Verification items for the finished model (mm, model axes). Face numbers are marked on the shaded views. Round coordinates to 2 decimals unless told otherwise and drop trailing zeros. Loops run counter-clockwise (first coordinate to the right, second up) from the corner with the lowest first, then second, coordinate; pieces in that order, holes last. Notation, with made-up numbers: (47.5, -24.5) - (98.5, -24.5) arc R31 ccw to (98.5, 4.5) - close; hole circle Ø7 at (-21.75, 87). An arc over 180 degrees is marked (long way). Use a Markdown table: item, result. Add a question column.
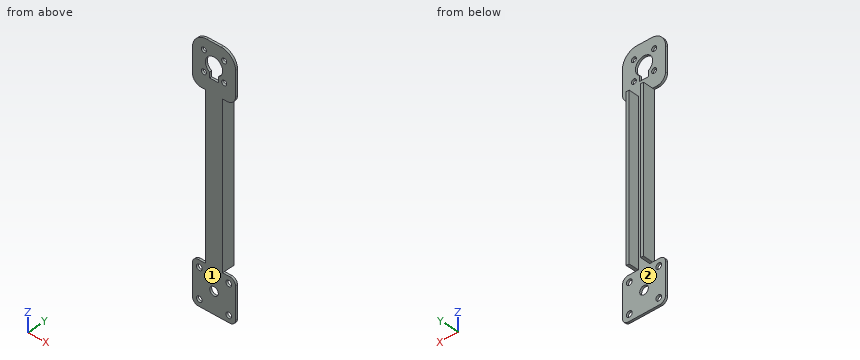
```python
from build123d import *

# Parameters (mm, degrees)
SKETCH_2_W           = 30
SKETCH_2_H           = 31
SKETCH_2_R           = 3
EXTRUDE_1_DEPTH      = 1.5
SKETCH_4_W           = 30
SKETCH_4_H           = 137
SKETCH_4_R           = 1.75
SKETCH_4_R_2         = 6
EXTRUDE_2_DEPTH      = 1.5
SKETCH_5_W           = 6
SKETCH_5_H           = 6
CUT_EXTRUDE_1_DEPTH  = 161.708587201
FILLET_7_R           = 10
CUT_EXTRUDE_2_DEPTH  = 161.708587201
FILLET_10_R          = 6
EXTRUDE_START        = -1.5
SKETCH_7_W           = 30
SKETCH_7_H           = 30
SKETCH_7_R           = 3
SKETCH_7_R_2         = 2
EXTRUDE_3_DEPTH      = 1.5
FILLET_12_R          = 4
EXTRUDE_4_DEPTH      = 7
EXTRUDE_4_DEPTH_BACK = 1.5
SKETCH_8_W           = 2
SKETCH_8_H           = 112


with BuildPart() as part:
    # 草图2 → 凸台-拉伸1 (new body)
    with BuildSketch(Plane(origin=(0, 0, 0), x_dir=(1, 0, 0), z_dir=(0, 1, 0))):
        with Locations((0, -7.5)):
            Rectangle(SKETCH_2_W, SKETCH_2_H)
        with Locations(Location((0, 0, 0), (0, 0, 270))):
            Circle(SKETCH_2_R, mode=Mode.SUBTRACT)
    extrude(amount=EXTRUDE_1_DEPTH)

    # 草图4 → 凸台-拉伸2 (add)
    with BuildSketch(Plane(origin=(0, 1.5, 0), x_dir=(1, 0, 0), z_dir=(0, 1, 0))):
        with Locations((0, -91.5)):
            Rectangle(SKETCH_4_W, SKETCH_4_H)
        with Locations(Location((7.071067812, -137.928932188, 0), (0, 0, 270))):
            Circle(SKETCH_4_R, mode=Mode.SUBTRACT)
        with Locations(Location((-7.071067812, -152.071067812, 0), (0, 0, 270))):
            Circle(SKETCH_4_R, mode=Mode.SUBTRACT)
        with Locations(Location((-7.071067812, -137.928932188, 0), (0, 0, 270))):
            Circle(SKETCH_4_R, mode=Mode.SUBTRACT)
        with Locations(Location((7.071067812, -152.071067812, 0), (0, 0, 270))):
            Circle(SKETCH_4_R, mode=Mode.SUBTRACT)
        with Locations(Location((0, -145, 0), (0, 0, 270))):
            Circle(SKETCH_4_R_2, mode=Mode.SUBTRACT)
    extrude(amount=-EXTRUDE_2_DEPTH)

    # 草图5 → 切除-拉伸1 (cut, through all)
    with BuildSketch(Plane(origin=(0, 1.5, 0), x_dir=(1, 0, 0), z_dir=(0, 1, 0))):
        with Locations((0, -139)):
            Rectangle(SKETCH_5_W, SKETCH_5_H)
    extrude(amount=-CUT_EXTRUDE_1_DEPTH, mode=Mode.SUBTRACT)

    # 圆角7
    fillet_7_edges = [part.edges().sort_by_distance(p)[0] for p in [
        (-15, 0.75, 160),
        (15, 0.75, 160),
    ]]
    fillet(fillet_7_edges, radius=FILLET_7_R)

    # 草图6 → 切除-拉伸2 (cut, through all)
    with BuildSketch(Plane(origin=(0, 1.5, 0), x_dir=(1, 0, 0), z_dir=(0, 1, 0))):
        Polygon((-8, 8), (-8, -8), (-4, -8), (-4, -127), (-8, -127), (-15, -127), (-15, 8), align=None)
        Polygon((15, 8), (8, 8), (8, -8), (4, -8), (4, -127), (8, -127), (15, -127), align=None)
    extrude(amount=-CUT_EXTRUDE_2_DEPTH, mode=Mode.SUBTRACT)

    # 圆角10
    fillet_10_edges = [part.edges().sort_by_distance(p)[0] for p in [
        (-15, 0.75, 127),
        (15, 0.75, 127),
    ]]
    fillet(fillet_10_edges, radius=FILLET_10_R)

    # 草图7 → 凸台-拉伸3 (add)
    with BuildSketch(Plane(origin=(0, 1.5, 0), x_dir=(1, 0, 0), z_dir=(0, 1, 0)).offset(EXTRUDE_START)):
        Rectangle(SKETCH_7_W, SKETCH_7_H)
        with Locations(Location((0, 0, 0), (0, 0, 270))):
            Circle(SKETCH_7_R, mode=Mode.SUBTRACT)
        with Locations(Location((-10.253048327, 10.253048327, 0), (0, 0, 270))):
            Circle(SKETCH_7_R_2, mode=Mode.SUBTRACT)
        with Locations(Location((10.253048327, 10.253048327, 0), (0, 0, 270))):
            Circle(SKETCH_7_R_2, mode=Mode.SUBTRACT)
        with Locations(Location((-10.253048327, -10.253048327, 0), (0, 0, 270))):
            Circle(SKETCH_7_R_2, mode=Mode.SUBTRACT)
        with Locations(Location((10.253048327, -10.253048327, 0), (0, 0, 270))):
            Circle(SKETCH_7_R_2, mode=Mode.SUBTRACT)
    extrude(amount=EXTRUDE_3_DEPTH)

    # 圆角12
    fillet_12_edges = [part.edges().sort_by_distance(p)[0] for p in [
        (15, 0.75, 15),
        (15, 0.75, -15),
        (-15, 0.75, 15),
        (-15, 0.75, -15),
    ]]
    fillet(fillet_12_edges, radius=FILLET_12_R)

    # 草图8 → 凸台-拉伸4 (add, two sides: drawn at the far end of the back side and taken through both)
    with BuildSketch(Plane(origin=(0, 1.5, 0), x_dir=(1, 0, 0), z_dir=(0, 1, 0)).offset(-EXTRUDE_4_DEPTH_BACK)):
        with Locations((-5, -71)):
            Rectangle(SKETCH_8_W, SKETCH_8_H)
        with Locations((5, -71)):
            Rectangle(SKETCH_8_W, SKETCH_8_H)
    extrude(amount=EXTRUDE_4_DEPTH + EXTRUDE_4_DEPTH_BACK)


solid = part.part
```
Q1. Go/stop test with flat-tipped pins: pin 1 Ø4.5 at (x, z) = (7.07, 137.93) entering from +Y; pin 2 Ø2 at (y, z) = (4, 86) entering from +X; pin 3 Ø3 at (y, z) = (3, 122.5) entering from -X. Record where each tip stops, or that it passes through.
Q2. Section check A-A on y = 3.5. Record the cut outline in (x, z), plus the area to 3 significant figures.
Q3. Thickness scan on line 1 along X through (y, z) = (7, 90); line 2 along Z through (x, y) = (-9, 1); line 3 along Y through (x, z) = (-9, 130). Record the ranges inside material, lowest first.
Q4. Section check B-B on x = 0. Record the cut outline in (y, z).
Q5. Section check C-C on z = 145. Record the cut outline in (x, y).
Q6. Section check D-D on z = 74.5. Record the cut outline in (x, y).
Q7. Release check for a two-part mould opening along X. For the marked faces 1 and 2 record: +X half, -X half, draft (parallel to the pull), parting line (faces both ways), or undercut.
Determined:
| question | item | result |
|---|---|---|
| 1 | pin 1 | stops at y = 1.5 |
| 1 | pin 2 | stops at x = 6 |
| 1 | pin 3 | stops at x = -6 |
| 2 | outline | (-6, 15) - (-4, 15) - (-4, 127) - (-6, 127) - close; (4, 15) - (6, 15) - (6, 127) - (4, 127) - close |
| 2 | area | 448 mm² |
| 3 | line 1 | x = -6 to -4, 4 to 6 |
| 3 | line 2 | z = -15 to -11.81, -8.69 to 8.69, 11.81 to 15, 127 to 159.17 |
| 3 | line 3 | y = 0 to 1.5 |
| 4 | outline | (0, -15) - (1.5, -15) - (1.5, -3) - (0, -3) - close; (0, 3) - (1.5, 3) - (1.5, 136) - (0, 136) - close; (0, 151) - (1.5, 151) - (1.5, 160) - (0, 160) - close |
| 5 | outline | (-15, 0) - (-6, 0) - (-6, 1.5) - (-15, 1.5) - close; (6, 0) - (15, 0) - (15, 1.5) - (6, 1.5) - close |
| 6 | outline | (-6, 0) - (6, 0) - (6, 8.5) - (4, 8.5) - (4, 1.5) - (-4, 1.5) - (-4, 8.5) - (-6, 8.5) - close |
| 7 | face 1 | draft |
| 7 | face 2 | undercut |
